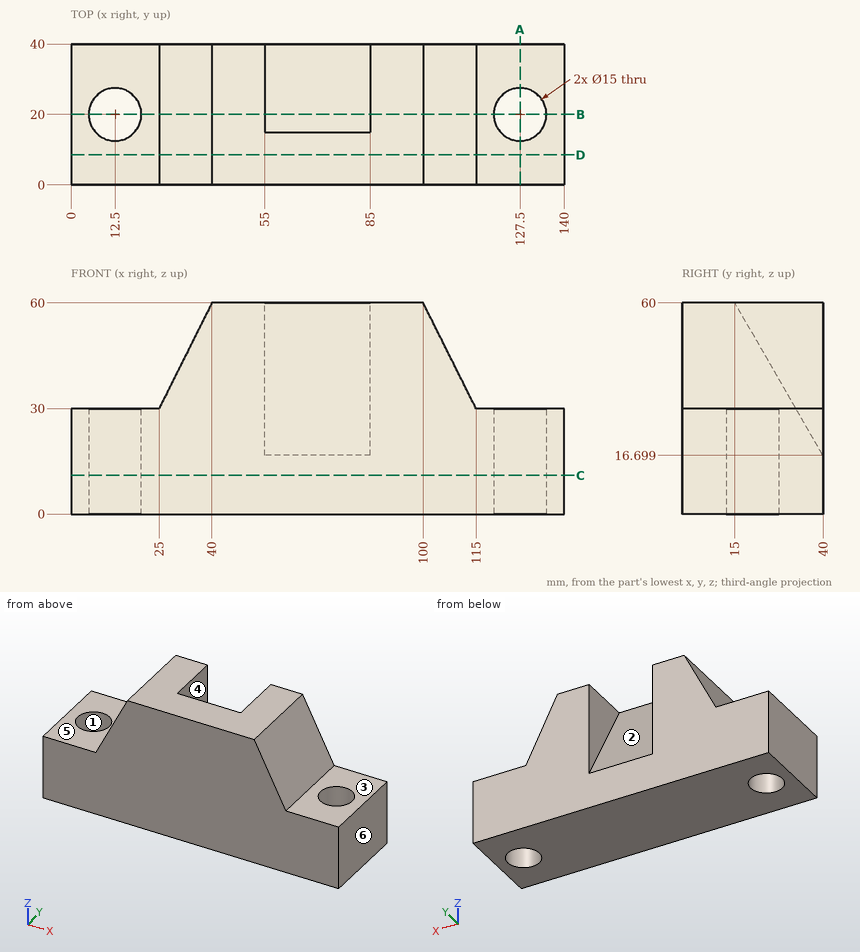
Answer from the drawing. Dimensions are ordinates in mm from the lowest x, y and z of the part. A direction names the side the tool comes from. Round coordinates to 2 decimals unless told otherwise and drop trailing zeros. Loops run counter-clockwise (first coordinate to the right, second up) from the corner with the lowest first, then second, coordinate; pieces in that order, holes last. Notation, with made-up numbers: (-21.5, -2.5) - (12.5, -2.5) arc R16 cw to (12.5, 28.5) - close; hole circle Ø1 at (39, 19). An arc over 180 degrees is marked (long way). Return JSON: item names as keys, results as strings. Group by question number.
1. The part is cut by section A-A on x = 127.5. Determine the outline of the cut face in (y, z), then the cut area to 3 significant figures.
2. The mould has two halves that part along X. Classify the marked faces 4, 5 and 6: pulls with the +X half, pulls with the -X half, needs draft (parallel to the pull), parting line crosses it, or undercut.
3. The part is cut by section C-C on z = 11. Determine the outline of the cut face in (x, y), then the cut area to 3 significant figures.
4. Which of the six approach directions +Z, -Z, +X, -X, +Y, -Y give full straight-line access (tool end or side, diameter ignored) to the marked faces 1, 2 and 3?
5. The part is cut by section D-D on y = 8.5. Determine the outline of the cut face in (x, z), then the cut area to 3 significant figures.
6. The part is cut by section B-B on y = 20. Determine the outline of the cut face in (x, z), then the cut area to 3 significant figures.
7. Each of these flat-tipped pins is pushed along its axis until it touches: P1, Ø8, axis at x = 24, y = 21, coming from the +Z side; P2, Ø20, axis at x = 132.5, y = 19, coming from the +Z side; P3, Ø1.5, axis at y = 17.5, z = 37, coming from the +X side (1 decimal); P4, Ø13.5, axis at x = 12.5, y = 20, coming from the +Z side. Where does it stop, or does it pass through?
8. Consider probe 1 along Y at (x, z) = (12, 23); probe 2 along X at (y, z) = (19.5, 2); probe 3 along X at (y, z) = (14, 27). Determine where each line is inside the solid, lowest interval first.
Resolved:
{
 "1": {"outline": "(0, 0) - (12.5, 0) - (12.5, 30) - (0, 30) - close; (27.5, 0) - (40, 0) - (40, 30) - (27.5, 30) - close", "area": "750 mm²"},
 "2": {"face 4": "undercut", "face 5": "needs draft", "face 6": "pulls with the +X half"},
 "3": {"outline": "(0, 0) - (140, 0) - (140, 40) - (0, 40) - close; hole circle Ø15 at (12.5, 20); hole circle Ø15 at (127.5, 20)", "area": "5,250 mm²"},
 "4": {"face 1": "+Z, -Z", "face 2": "+Z, +Y", "face 3": "+Z, +X, +Y, -Y"},
 "5": {"outline": "(0, 0) - (140, 0) - (140, 30) - (115, 30) - (100, 60) - (40, 60) - (25, 30) - (0, 30) - close", "area": "6,450 mm²"},
 "6": {"outline": "(0, 0) - (5, 0) - (5, 30) - (0, 30) - close; (20, 0) - (120, 0) - (120, 30) - (115, 30) - (100, 60) - (85, 60) - (85, 51.34) - (55, 51.34) - (55, 60) - (40, 60) - (25, 30) - (20, 30) - close; (135, 0) - (140, 0) - (140, 30) - (135, 30) - close", "area": "5,290 mm²"},
 "7": {"P1": "stops at z = 36", "P2": "stops at z = 30", "P3": "stops at x = 111.9", "P4": "passes through"},
 "8": {"probe 1": "y = 0 to 12.52, 27.48 to 40", "probe 2": "x = 0 to 5.02, 19.98 to 120.02, 134.98 to 140", "probe 3": "x = 0 to 8, 17 to 123, 132 to 140"}
}
